Can you work these out from the model? Positions are in its coordinate system, mm. Face numbers are marked on the shaded views. A direction names the side the tool comes from. Give positions to 0.01 mm unless a question says otherwise; leave off trailing zeros. Write each loop counter-clockwise with the first axis right and the second up, starting at its lowest first coordinate (ties: lowest second). Pieces come first, ordered by that corner, then holes.
```python
from build123d import *

# Parameters (mm, degrees)
SKETCH1_R           = 35
BOSS_EXTRUDE1_DEPTH = 5
SKETCH4_R           = 3
CUT_EXTRUDE1_DEPTH  = 5
SKETCH5_R           = 10
BOSS_EXTRUDE2_DEPTH = 20
SKETCH6_R           = 4
CUT_EXTRUDE2_DEPTH  = 20


with BuildPart() as part:
    # Sketch1 → Boss-Extrude1 (new body)
    with BuildSketch(Plane.XY):
        Circle(SKETCH1_R)
    extrude(amount=BOSS_EXTRUDE1_DEPTH)

    # Sketch4 → Cut-Extrude1 (cut)
    with BuildSketch(Plane.XY.offset(5)):
        with Locations((0, 30)):
            Circle(SKETCH4_R)
        with Locations((30, 0)):
            Circle(SKETCH4_R)
        with Locations((0, -30)):
            Circle(SKETCH4_R)
        with Locations((-30, 0)):
            Circle(SKETCH4_R)
    extrude(amount=-CUT_EXTRUDE1_DEPTH, mode=Mode.SUBTRACT)

    # Sketch5 → Boss-Extrude2 (add)
    with BuildSketch(Plane.XY.offset(5)):
        Circle(SKETCH5_R)
    extrude(amount=BOSS_EXTRUDE2_DEPTH)

    # Sketch6 → Cut-Extrude2 (cut)
    with BuildSketch(Plane.XY.offset(25)):
        Circle(SKETCH6_R)
    extrude(amount=-CUT_EXTRUDE2_DEPTH, mode=Mode.SUBTRACT)


solid = part.part
```
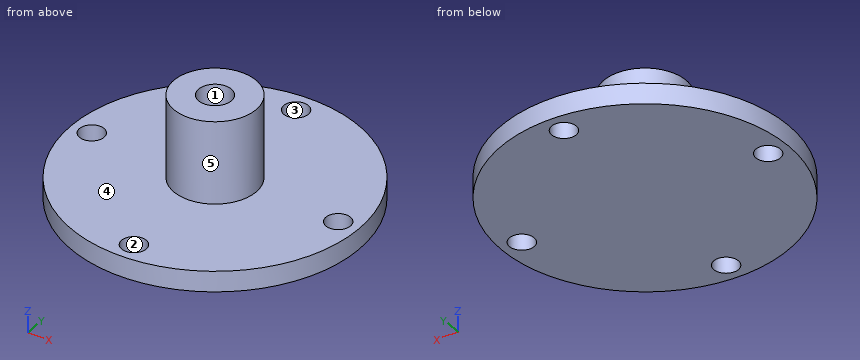
1) Suppose I cut it at D-D on x = -30. Write out the boundary of the cut face in (y, z), plus the area to 3 significant figures.
Values follow:
outline: (-18.03, 0) - (-3, 0) - (-3, 5) - (-18.03, 5) - close; (3, 0) - (18.03, 0) - (18.03, 5) - (3, 5) - close
area: 150 mm2
2) For the marked faces 1 and 2, which set-ups out of +Z, -Z, +X, -X, +Y, -Y let a thin tool reach every point of the face, with its end or its side?
Values follow:
face 1: +Z
face 2: +Z, -Z
3) Suppose I cut it at C-C on z = 12.75. Write out the boundary of the cut face in (x, y).
Values follow:
outline: circle Ø20 at (0, 0); hole circle Ø8 at (0, 0)
4) For pin 1 Ø10 at (x, y) = (10, 17) entering from +Z; pin 2 Ø5 at (x, z) = (-18, 5) entering from -Y; pin 3 Ø1.5 at (y, z) = (-0.5, 14.5) entering from +X, each with a flat end and sliding along its axis, tell me the tip position at first contact or that it passes through.
Values follow:
pin 1: stops at z = 5
pin 2: stops at y = -31.38
pin 3: stops at x = 10
5) Please list where these lines run through material, in increasing order: L1, parallel to Y at x = 0, z = 1.75; L2, parallel to Y at x = 0, z = 9; L3, parallel to Z at x = -13, y = -25.
Values follow:
L1: y = -35 to -33, -27 to 27, 33 to 35
L2: y = -10 to -4, 4 to 10
L3: z = 0 to 5
6) If we mould it in two halves opening along X, with no side actions, what happens to the marked faces 3, 4 and 5? For each: +X half, -X half, draft (parallel to the pull), parting line (faces both ways), or undercut.
Values follow:
face 3: undercut
face 4: draft
face 5: parting line
7) Suppose I cut it at A-A on x = 0. Write out the boundary of the cut face in (y, z).
Values follow:
outline: (-35, 0) - (-33, 0) - (-33, 5) - (-35, 5) - close; (-27, 0) - (27, 0) - (27, 5) - (10, 5) - (10, 25) - (4, 25) - (4, 5) - (-4, 5) - (-4, 25) - (-10, 25) - (-10, 5) - (-27, 5) - close; (33, 0) - (35, 0) - (35, 5) - (33, 5) - close
